from build123d import *

# Parameters (mm, degrees)
F0_R     = 1.225
F1_DEPTH = 2.75
F2_DEPTH = 25
F3_W     = 2.7319499059
F3_H     = 6.5613500774
F3_W_2   = 2.5918500032
F3_W_3   = 2.8168536527
F3_H_2   = 7.1630705833
F3_W_4   = 2.5843745833
F4_DEPTH = 5


with BuildPart() as f1:
    # F0 (on Front) → F1 (new body, symmetric)
    with BuildSketch(Plane.XZ):
        with BuildLine():
            ThreePointArc((-2.75, -20.05), (0, -22.8), (2.75, -20.05))
            Line((2.75, -20.05), (2.75, 20.05))
            ThreePointArc((2.75, 20.05), (0, 22.8), (-2.75, 20.05))
            Line((-2.75, 20.05), (-2.75, -20.05))
        make_face()
        with Locations((0, -20.05)):
            Circle(F0_R, mode=Mode.SUBTRACT)
        with BuildLine():
            Line((-1.225, -11.175), (-1.225, 11.175))
            ThreePointArc((-1.225, 11.175), (0, 12.4), (1.225, 11.175))
            Line((1.225, 11.175), (1.225, -11.175))
            ThreePointArc((1.225, -11.175), (0, -12.4), (-1.225, -11.175))
        make_face(mode=Mode.SUBTRACT)
        with Locations((0, 20.05)):
            Circle(F0_R, mode=Mode.SUBTRACT)
    extrude(amount=F1_DEPTH, both=True)

    # F0 (on Front) → F2 (cut)
    with BuildSketch(Plane.XZ):
        with Locations((0, 20.05)):
            Circle(F0_R)
        with BuildLine():
            ThreePointArc((1.225, 11.175), (0, 12.4), (-1.225, 11.175))
            Line((-1.225, 11.175), (-1.225, -11.175))
            ThreePointArc((-1.225, -11.175), (0, -12.4), (1.225, -11.175))
            Line((1.225, -11.175), (1.225, 11.175))
        make_face()
        with Locations((0, -20.05)):
            Circle(F0_R)
    extrude(amount=-F2_DEPTH, mode=Mode.SUBTRACT)

    # F3 (on Right) → F4 (cut, symmetric)
    with BuildSketch(Plane.YZ):
        with Locations((-2.8040870675, 20.3422307968)):
            Rectangle(F3_W, F3_H)
        with Locations((2.7298625791, 20.3422307968)):
            Rectangle(F3_W_2, F3_H)
        with Locations((-2.8399268263, -19.7806989431)):
            Rectangle(F3_W_3, F3_H_2)
        with Locations((2.7236872916, -19.7806989431)):
            Rectangle(F3_W_4, F3_H_2)
    extrude(amount=F4_DEPTH, both=True, mode=Mode.SUBTRACT)


solid = f1.part
Could you check a few things on this model? Use its own coordinates, in mm. A direction names the side the tool comes from. Round coordinates to 2 decimals unless told otherwise and drop trailing zeros. Order: outer loops, then holes, each group sorted by start corner. A loop starts at its lowest first (then second) coordinate and runs counter-clockwise, first axis right, second up.
(1) Imagine slicing it at C-C (y = 2.1). Write out the boundary of the cut face in (x, z) (3 decimals), plus the area to 3 significant figures.
Response values:
outline: (-2.75, -16.199) - (2.75, -16.199) - (2.75, 17.062) - (-2.75, 17.062) - close; hole (-1.225, -11.175) arc R1.225 ccw to (1.225, -11.175) - (1.225, 11.175) arc R1.225 ccw to (-1.225, 11.175) - close
area: 123 mm2
(2) Which directions (+Z, -Z, +X, -X, +Y, -Y) give clear straight access to the entire face, cutting with the end or side of a thin tool? Please do faces 4 (the flat face through (-1, -1.431, -19)), 5 (the flat face through (0, 2, 17.062)), 6 (the cylindrical face through (0, 0, 12.4)).
Response values:
face 4: -Z, +X, -X, -Y
face 5: +Z, +X, -X, +Y
face 6: +Y, -Y
(3) Imagine slicing it at D-D (x = 2.1). Write out the boundary of the cut face in (y, z), plus the area to 3 significant figures.
Response values:
outline: (-2.75, -16.2) - (-1.43, -16.2) - (-1.43, -21.83) - (1.43, -21.83) - (1.43, -16.2) - (2.75, -16.2) - (2.75, 17.06) - (1.43, 17.06) - (1.43, 21.83) - (-1.44, 21.83) - (-1.44, 17.06) - (-2.75, 17.06) - close
area: 213 mm2
(4) Please list where these lines run through material, in increasing order: line 1 along Z through (x, y) = (0, 0.1) (3 decimals); line 2 along X through (y, z) = (-0.3, -20.05) (3 decimals); line 3 along Z through (x, y) = (0.35, 0.9).
Response values:
line 1: z = -22.8 to -21.275, -18.825 to -12.4, 12.4 to 18.825, 21.275 to 22.8
line 2: x = -2.75 to -1.225, 1.225 to 2.75
line 3: z = -22.78 to -21.22, -18.88 to -12.35, 12.35 to 18.88, 21.22 to 22.78
(5) I'm going to push flat-ended pins straight in: pin 1 (1.6 mm diameter, centred on x = 0, z = -18, fed in from +Y); pin 2 (2 mm diameter, centred on x = 2, y = 1.5, fed in from +Z); pin 3 (0.7 mm diameter, centred on x = 0, y = -2, fed in from +Z). Where does each tip first touch, or does it pass through?
Response values:
pin 1: stops at y = 1.43
pin 2: stops at z = 22.61
pin 3: stops at z = 17.06
(6) Imagine slicing it at B-B (z = 10.5). Write out the boundary of the cut face in (x, y) (3 decimals).
Response values:
outline: (-2.75, -2.75) - (-1.225, -2.75) - (-1.225, 2.75) - (-2.75, 2.75) - close; (1.225, -2.75) - (2.75, -2.75) - (2.75, 2.75) - (1.225, 2.75) - close
(7) Imagine slicing it at A-A (x = 0). Count the separate pieces of the cut face and the enclosed holes in it, plus the area to 3 significant figures.
Response values:
separate pieces: 4
enclosed holes: 0
area: 67.9 mm2
(8) If we mould it in two halves opening along Z, with no side actions, what happens to faces 1 (the flat face through (0, -2, 17.062)), 2 (the cylindrical face through (-0.266, 0.02, -21.246)), 3 (the flat face through (-2, 2.75, 1))? For each: released by +Z, released by -Z, zero draft, split by the parting line, or undercut.
Response values:
face 1: released by +Z
face 2: undercut
face 3: zero draft
